Check sheet for the drawn part. Datum: minimum x, y, z corner. Units: mm. Round coordinates to 2 decimals unless told otherwise and drop trailing zeros. Write each loop counter-clockwise with the first axis right and the second up, starting at its lowest first coordinate (ties: lowest second). Pieces come first, ordered by that corner, then holes. Notation, with made-up numbers: (8, 39) - (56, 39) arc R11 ccw to (56, 53) - close; hole circle Ø9 at (-29, 63.25). An arc over 180 degrees is marked (long way). Answer as a JSON object with one key per item and string values. Group by question number.
1) Thickness scan on line 1 (X direction, y = 6, z = 6.5); line 2 (Z direction, x = 23.5, y = 2.6); line 3 (Z direction, x = 23.5, y = 2.3). Record the ranges inside material, lowest first.
2) Go/stop test with flat-tipped pins: pin 1 Ø1.6 at (y, z) = (7, 3.5) entering from -X; pin 2 Ø1.5 at (x, y) = (12, 5) entering from -Z; pin 3 Ø2 at (x, z) = (25.5, 5) entering from +Y. Record where each tip stops, or that it passes through.
3) Section check C-C (x = 23.5). Enter the section's corners in (y, z), then the cut area to 3 significant figures.
4) Section check B-B (y = 3.93). Enter the section's corners in (x, z), then the cut area to 3 significant figures.
5) Section check A-A (z = 3.93). Enter the section's corners in (x, y), then the cut area to 3 significant figures.
6) Mould release check, pull along X, two halves, no side actions. Record for the marked faces 1, 2 and 3: +X half, -X half, draft (parallel to the pull), parting line (faces both ways), or undercut.
7) Section check D-D (x = 4). Enter the section's corners in (y, z).
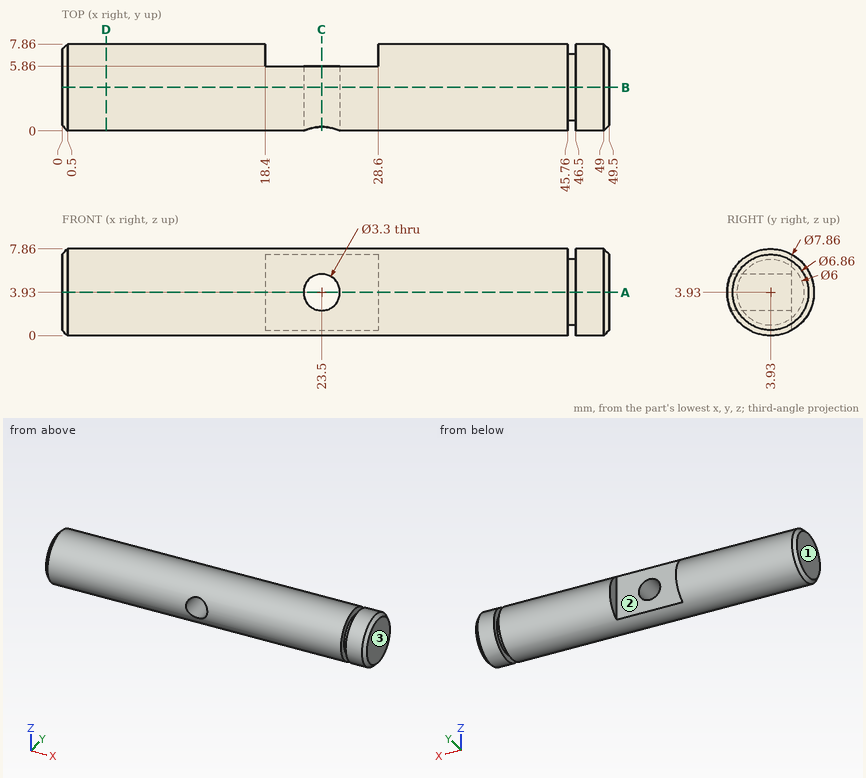
Returned:
{
 "1": {"line 1": "0 to 18.4, 28.6 to 45.76, 46.5 to 49.5", "line 2": "0.23 to 2.28, 5.58 to 7.63", "line 3": "0.35 to 2.28, 5.58 to 7.51"},
 "2": {"pin 1": "x = 0", "pin 2": "z = 0.01", "pin 3": "y = 5.86"},
 "3": {"outline": "(0.36, 2.28) arc R3.93 ccw to (5.86, 0.51) - (5.86, 2.28) - close; (0.36, 5.58) - (5.86, 5.58) - (5.86, 7.35) arc R3.93 ccw to start", "area": "19.9 mm2"},
 "4": {"outline": "(0, 0.5) - (0.5, 0) - (45.76, 0) - (45.76, 0.93) - (46.5, 0.93) - (46.5, 0) - (49, 0) - (49.5, 0.5) - (49.5, 7.36) - (49, 7.86) - (46.5, 7.86) - (46.5, 6.93) - (45.76, 6.93) - (45.76, 7.86) - (0.5, 7.86) - (0, 7.36) - close; hole circle Ø3.3 at (23.5, 3.93)", "area": "379 mm2"},
 "5": {"outline": "(0, 0.5) - (0.5, 0) - (21.85, 0) - (21.85, 5.86) - (18.4, 5.86) - (18.4, 7.86) - (0.5, 7.86) - (0, 7.36) - close; (25.15, 0) - (45.76, 0) - (45.76, 0.93) - (46.5, 0.93) - (46.5, 0) - (49, 0) - (49.5, 0.5) - (49.5, 7.36) - (49, 7.86) - (46.5, 7.86) - (46.5, 6.93) - (45.76, 6.93) - (45.76, 7.86) - (28.6, 7.86) - (28.6, 5.86) - (25.15, 5.86) - close", "area": "347 mm2"},
 "6": {"face 1": "-X half", "face 2": "undercut", "face 3": "+X half"},
 "7": {"outline": "circle Ø7.86 at (3.93, 3.93)"}
}
